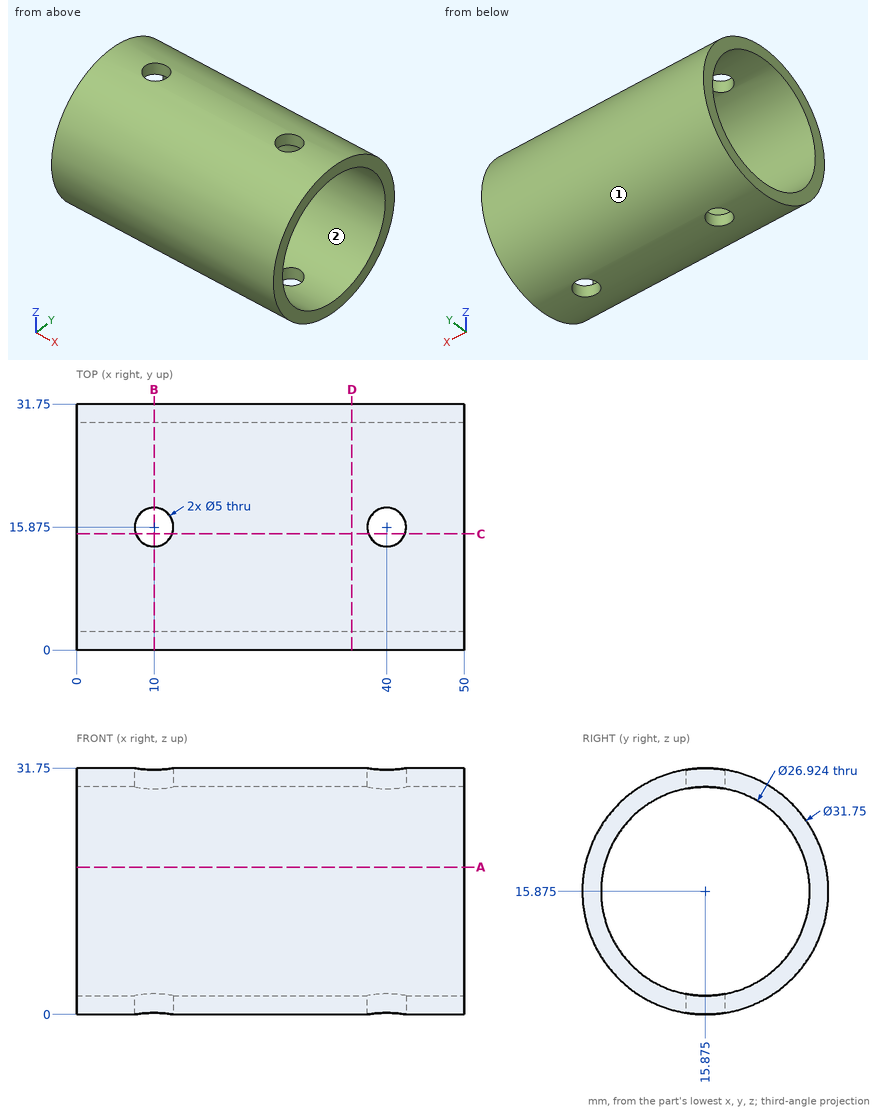
Job drawing, mm, ordinate dimensions from the low corner. One solid piece. Coordinates: 2 decimals unless noted, no trailing zeros. Write each loop counter-clockwise with the first axis right and the second up, starting at its lowest first coordinate (ties: lowest second). Pieces come first, ordered by that corner, then holes.
Item 1: Mould opens along Y. For the marked faces 1 and 2 say: released by +Y, released by -Y, zero draft, split by the parting line, or undercut.
Item 2: Pin check, flat tips, straight feed: pin 1 (3 mm diameter, centred on x = 20, z = 8.5, fed in from +Y); pin 2 (1.5 mm diameter, centred on x = 42.5, z = 8, fed in from +Y); pin 3 (1.5 mm diameter, centred on x = 19.5, z = 17, fed in from +Y). Stop position of each tip, or through.
Item 3: Slice it at B-B (x = 10). Write the cut outline in (y, z) (3 decimals).
Item 4: Slice it at A-A (z = 19). Write the cut outline in (x, y), and give its area (3 significant figures).
Item 5: Slice it at D-D (x = 35.5). Write the cut outline in (y, z) (3 decimals), and give its area (3 significant figures).
Item 6: Probe line 1 (Y direction, x = 32, z = 8); line 2 (Z direction, x = 12, y = 23); line 3 (Z direction, x = 20.5, y = 27). List the from-to ranges inside material, lowest first.
Item 7: Slice it at C-C (y = 15). Write the cut outline in (x, z).
Results found:
1. face 1: split by the parting line
1. face 2: undercut
2. pin 1: stops at y = 30.62
2. pin 2: stops at y = 30.06
2. pin 3: stops at y = 31.75
3. outline: (13.375, 0.198) - (13.375, 2.647) arc R13.462 cw to (13.375, 29.103) - (13.375, 31.552) arc R15.875 ccw to start; (18.375, 0.198) arc R15.875 ccw to (18.375, 31.552) - (18.375, 29.103) arc R13.462 cw to (18.375, 2.647) - close
4. outline: (0, 0.31) - (50, 0.31) - (50, 2.78) - (0, 2.78) - close; (0, 28.97) - (50, 28.97) - (50, 31.44) - (0, 31.44) - close
4. area: 247 mm2
5. outline: circle Ø31.75 at (15.875, 15.875); hole circle Ø26.924 at (15.875, 15.875)
5. area: 222 mm2
6. line 1: y = 2.09 to 4.96, 26.79 to 29.66
6. line 2: z = 1.69 to 4.45, 27.3 to 30.06
6. line 3: z = 4.55 to 8.29, 23.46 to 27.2
7. outline: (0, 0.02) - (7.66, 0.02) - (7.66, 2.44) - (0, 2.44) - close; (0, 29.31) - (7.66, 29.31) - (7.66, 31.73) - (0, 31.73) - close; (12.34, 0.02) - (37.66, 0.02) - (37.66, 2.44) - (12.34, 2.44) - close; (12.34, 29.31) - (37.66, 29.31) - (37.66, 31.73) - (12.34, 31.73) - close; (42.34, 0.02) - (50, 0.02) - (50, 2.44) - (42.34, 2.44) - close; (42.34, 29.31) - (50, 29.31) - (50, 31.73) - (42.34, 31.73) - close
